For this review, take the finished solid that the model builds, in its own axes (mm). Face numbers are marked on the shaded views. Coordinates: 2 decimals unless noted, no trailing zeros. Order: outer loops, then holes, each group sorted by start corner. A loop starts at its lowest first (then second) coordinate and runs counter-clockwise, first axis right, second up. Notation, with made-up numbers: M 68.5,62 L 114.5,62 A27 ccw 114.5,92 Z; hole C -20,-25 d7. An arc over 180 degrees is marked long. Use CSV: the item, a comma, the result in double quotes.
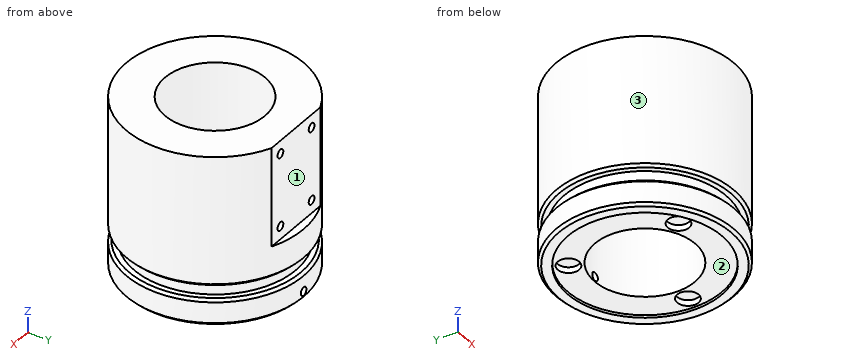
Autodesk Inventor part; units mm, degrees
ref_plane "Plano de trabalho1" through (0, 0, 65) normal (0, 0, 1) x (1, 0, 0)
ref_plane "Plano de trabalho2" through (-13.8302, 31.06, 65) normal (0, 1, 0) x (1, 0, 0)
ref_plane "Plano de trabalho3" through (0, 0, 1) normal (0, 0, -1) x (-1, 0, 0)
sketch "Esboço2" plane through (0, 0, 0) normal (0, 1, 0) x (-1, 0, 0)
  line L0 (0, 0) -> (-19.2, 0) construction
  line L1 (-34, 1) -> (-34, 9)
  line L2 (-33, 10) -> (-31, 10)
  line L3 (-31, 10) -> (-31, 15)
  line L4 (-31, 15) -> (-33, 15)
  line L5 (-34, 16) -> (-34, 65)
  line L6 (0, 0) -> (0, 69.2361) construction
  line L7 (-34, 65) -> (-19.2, 65)
  line L8 (-19.2, 0) -> (-19.2, 1)
  line L9 (-19.2, 1) -> (-29.5, 1)
  line L10 (-29.5, 1) -> (-29.5, 0)
  line L11 (-29.5, 0) -> (-33, 0)
  line L12 (-19.2, 1) -> (-19.2, 65)
  line L13 (-34, 16) -> (-33, 15)
  line L14 (-34, 9) -> (-33, 10)
  line L15 (-34, 1) -> (-33, 0)
  point P0 (-34, 0)
  point P1 (-34, 10)
  point P2 (-34, 15)
  dimension "d1" = 19.2
  dimension "d6" = 14.8
  dimension "d7" = 10
  dimension "d8" = 3
  dimension "d9" = 5
  dimension "d11" = 50
  dimension "d14" = 1
  dimension "d15" = 10.3
  dimension "d16" = 1
  dimension "d17" = 1
  dimension "d18" = 1
  dimension "d19" = 1
  dimension "d20" = 1
  dimension "d21" = 1
revolve "Revolução1" add sketch "Esboço2" angle 360 about axis through (0, 0, 0) along (0, 0, 1)
ref_plane "Plano de trabalho1" through (0, 0, 65) normal (0, 0, 1) x (1, 0, 0)
sketch "Esboço3" plane through (0, 0, 65) normal (0, 0, 1) x (1, 0, 0)
  line L0 (0, 0) -> (0, 19.06) construction
  line L1 (0, 19.06) -> (0, 31.06) construction
  line L2 (0, 31.06) -> (33, 31.06) construction
  line L3 (33, 31.06) -> (33, 44.9163)
  line L4 (33, 44.9163) -> (-33, 44.9163)
  line L5 (-33, 44.9163) -> (-33, 31.06)
  line L6 (-33, 31.06) -> (33, 31.06)
  dimension "d30" = 12
  dimension "d31" = 19.06
extrude "Extrusão1" cut sketch "Esboço3" against normal blind 38
ref_plane "Plano de trabalho2" through (-13.8302, 31.06, 65) normal (0, 1, 0) x (1, 0, 0)
sketch "Esboço5" plane through (-13.8302, 31.06, 65) normal (0, 1, 0) x (1, 0, 0)
  line L0 (0, 0) -> (0, 38)
  line L1 (27.6605, 0) -> (0, 0)
  line L2 (27.6605, 38) -> (27.6605, 0)
  line L3 (5, 5) -> (5, 33)
  line L4 (5, 33) -> (22.6605, 33)
  line L5 (22.6605, 33) -> (22.6605, 5)
  line L6 (22.6605, 5) -> (5, 5)
  line L7 (27.6605, 38) -> (0, 38)
  point P0 (13.8302, 65)
  dimension "d33" = 5
hole "Furo1" at (8.8302, 31.06, 60) at (8.8302, 31.06, 32) at (-8.8302, 31.06, 32) at (-8.8302, 31.06, 60) direction (0, -1, 0) diameter 3.242 depth 8 tip angle 118
ref_plane "Plano de trabalho3" through (0, 0, 1) normal (0, 0, -1) x (-1, 0, 0)
sketch "Esboço7" plane through (0, 0, 1) normal (0, 0, -1) x (-1, 0, 0)
  circle A0 centre (0, 0) radius 19.2 construction
  circle A1 centre (0, 0) radius 29.2679 construction
  circle A2 centre (0, 0) radius 19.2
  line L0 (-19.2, 0) -> (-24.367, 0) construction
  circle A3 centre (-24.367, 0) radius 4.1
  circle A4 centre (12.1835, -21.1024) radius 4.1
  circle A5 centre (12.1835, 21.1024) radius 4.1
  dimension "d42" = 5.167
  dimension "d43" = 8.2
  dimension "d46" = 360
extrude "Extrusão2" cut sketch "Esboço7" against normal blind 2.2 contours A3 | A4 | A5
ref_plane "Plano de trabalho4" through (-13.8302, 31.06, 65) normal (0, 1, 0) x (1, 0, 0)
ref_plane "Plano de trabalho5" through (0, 34, 27) normal (0, 1, 0) x (-1, 0, 0)
sketch "Esboço10" plane through (0, 34, 27) normal (0, 1, 0) x (-1, 0, 0)
  line L0 (-13.8302, 0) -> (13.8302, 0)
  line L1 (0, 0) -> (0, -27) construction
  line L2 (0, -27) -> (0, -24) construction
  dimension "d53" = 3
hole "Furo2" at (0, 34, 3) direction (0, -1, 0) diameter 3.2 depth 17.2 tip angle 118
properties part number "bocal_de_aquecimento" material "Alumínio 6061"
Item 1: Add section B-B on x = 0. State how many separate pieces and enclosed holes the cut face has, and give its area (3 significant figures).
Solutions:
separate pieces,"3"
enclosed holes,"0"
area,"1,710 mm^2"
Item 2: To check wall thickness, follow line 1 along Y through (x, z) = (-0.5, 48); line 2 along X through (y, z) = (29, 32); line 3 along Z through (x, y) = (25, 3.5). State the ranges of each line that lie inside material, in increasing order. Write a range as [from, to].
Solutions:
line 1,"[-34, -19.19], [19.19, 31.06]"
line 2,"[-17.75, -10.45], [-7.21, 7.21], [10.45, 17.75]"
line 3,"[3.2, 65]"
Item 3: Draft analysis for pull direction Y (two halves, no side actions). For the marked faces 1, 2 and 3, state which applies: released by +Y, released by -Y, zero draft, split by the parting line, or undercut.
Solutions:
face 1,"released by +Y"
face 2,"undercut"
face 3,"split by the parting line"
Item 4: Add section D-D on z = 44. State the section outline as (x, y) points, and give its area (3 significant figures).
Solutions:
outline,"M -13.83,31.06 A34 ccw long 13.83,31.06 Z; hole C 0,0 d38.4"
area,"2,420 mm^2"
Item 5: Clearance check with flat-ended pins moving along their axes: pin 1 Ø1.9 at (x, z) = (8.83, 32) entering from -Y; pin 2 Ø1.9 at (x, z) = (0, 3) entering from +Y; pin 3 Ø4 at (x, y) = (26, 1.5) entering from -Z. State where each tip first meets the part, or that it passes through.
Solutions:
pin 1,"y = -33.07"
pin 2,"y = -19.18"
pin 3,"z = 1"
Item 6: Add section C-C on z = 6. State the section outline as (x, y) points, and give its area (3 significant figures).
Solutions:
outline,"C 0,0 d68; hole C 0,0 d38.4"
area,"2,470 mm^2"
